Part print with two shaded views. Sizes in mm from the minimum x, y, z corner. A direction names the side the tool comes from. Give positions to 0.01 mm unless a question says otherwise; leave off trailing zeros. Write each loop counter-clockwise with the first axis right and the second up, starting at its lowest first coordinate (ties: lowest second). Pieces come first, ordered by that corner, then holes. Notation, with made-up numbers: (61.5, -34) - (90.5, -34) arc R10 ccw to (90.5, -26) - close; hole circle Ø5 at (68.5, -8). An arc over 180 degrees is marked (long way). Answer as a JSON object with one key per item and string values.
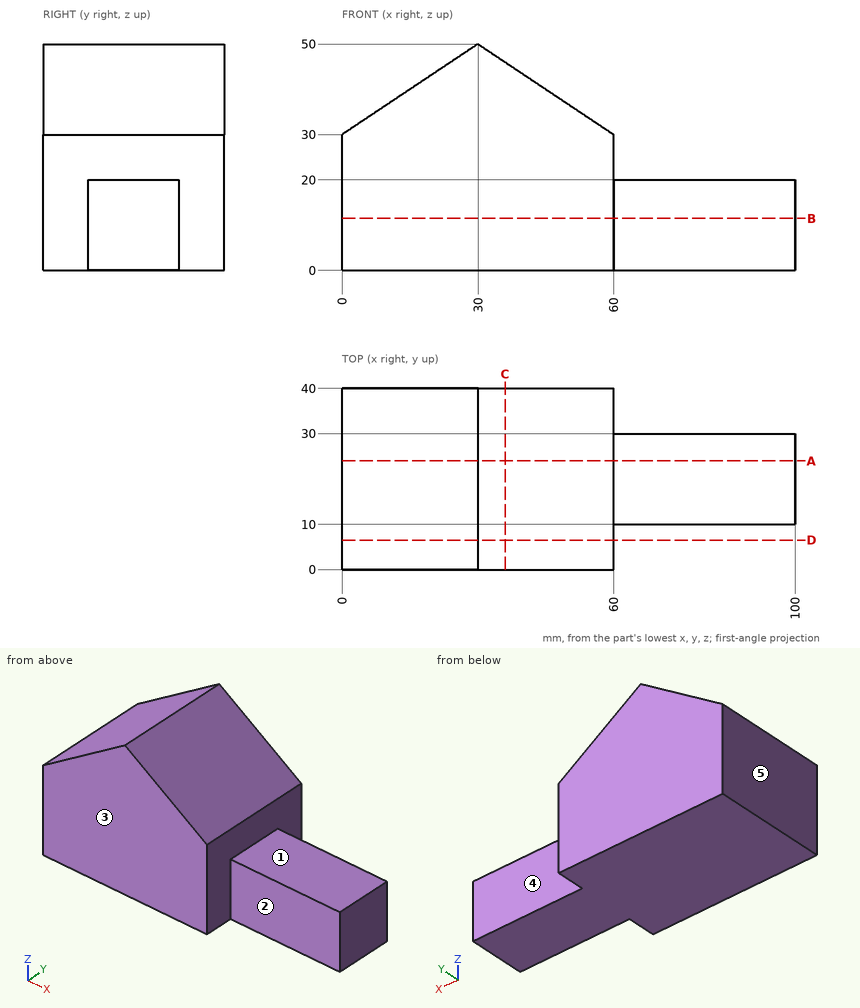
(1) Saw through at C-C, the plane x = 36. Give the cut face in (y, z).
Answer key:
{"outline": "(0, 0) - (40, 0) - (40, 46) - (0, 46) - close"}
(2) 3-axis set-ups, long thin cutter, end or side, ignore diameter. For the marked faces 1, 2, 3, 4 and 5: which of +Z, -Z, +X, -X, +Y, -Y reach the whole face in a straight line?
Answer key:
{"face 1": "+Z, +X, +Y, -Y", "face 2": "+Z, -Z, +X, -Y", "face 3": "+Z, -Z, +X, -X, -Y", "face 4": "+Z, -Z, +X, +Y", "face 5": "+Z, -Z, -X, +Y, -Y"}
(3) Saw through at D-D, the plane y = 6.5. Give the cut face in (x, z).
Answer key:
{"outline": "(0, 0) - (60, 0) - (60, 30) - (30, 50) - (0, 30) - close"}
(4) Saw through at B-B, the plane z = 11.5. Give the cut face in (x, y), and give its area (3 significant figures).
Answer key:
{"outline": "(0, 0) - (60, 0) - (60, 10) - (100, 10) - (100, 30) - (60, 30) - (60, 40) - (0, 40) - close", "area": "3,200 mm²"}
(5) Saw through at A-A, the plane y = 24. Give the cut face in (x, z), and give its area (3 significant figures).
Answer key:
{"outline": "(0, 0) - (100, 0) - (100, 20) - (60, 20) - (60, 30) - (30, 50) - (0, 30) - close", "area": "3,200 mm²"}
(6) Probe L1, parallel to X at y = 33.5, z = 14.5; L2, parallel to Z at x = 88, y = 20; L3, parallel to Y at x = 94.5, z = 5.5. List the from-to ranges inside material, lowest first. Write a range as [from, to].
Answer key:
{"L1": "x = [0, 60]", "L2": "z = [0, 20]", "L3": "y = [10, 30]"}
(7) Flat gauge pins, fed straight in: P1, Ø6, axis at x = 76, y = 32, coming from the +Z side; P2, Ø16, axis at x = 90, z = 7.5, coming from the +Y side; P3, Ø1, axis at y = 14.5, z = 38, coming from the +X side. Where does each tip first touch, or does it go through?
Answer key:
{"P1": "stops at z = 20", "P2": "stops at y = 30", "P3": "stops at x = 48.75"}
